from build123d import *

# Parameters (mm, degrees)
SKETCH_1_W          = 21
SKETCH_1_H          = 66
EXTRUDE_1_DEPTH     = 1.1
SKETCH_2_R          = 3
CUT_EXTRUDE_1_DEPTH = 35.647655043
SKETCH_3_W          = 21
SKETCH_3_H          = 66
SKETCH_3_W_2        = 12
SKETCH_3_H_2        = 51
EXTRUDE_2_DEPTH     = 3.9
SKETCH_4_R          = 1.9
SKETCH_4_R_2        = 1
CUT_EXTRUDE_2_DEPTH = 3
SKETCH_4_2_R        = 1
CUT_EXTRUDE_3_DEPTH = 35.989284074


with BuildPart() as part:
    # 草图1 → 凸台-拉伸1 (new body)
    with BuildSketch(Plane(origin=(0, 0, 0), x_dir=(1, 0, 0), z_dir=(0, 1, 0))):
        Rectangle(SKETCH_1_W, SKETCH_1_H)
    extrude(amount=EXTRUDE_1_DEPTH)

    # 草图2 → 切除-拉伸1 (cut, through all)
    with BuildSketch(Plane(origin=(0, 0, 0), x_dir=(-1, 0, 0), z_dir=(0, -1, 0))):
        with Locations(Location((-1.458325738, -20.003345868, 0), (0, 0, 90))):
            Circle(SKETCH_2_R)
        with Locations(Location((-1.786068296, -0.006031428, 0), (0, 0, 90))):
            Circle(SKETCH_2_R)
        with Locations(Location((-2.113810854, 19.991283012, 0), (0, 0, 90))):
            Circle(SKETCH_2_R)
    extrude(amount=-CUT_EXTRUDE_1_DEPTH, mode=Mode.SUBTRACT)

    # 草图3 → 凸台-拉伸2 (add)
    with BuildSketch(Plane(origin=(0, 1.1, 0), x_dir=(1, 0, 0), z_dir=(0, 1, 0))):
        Rectangle(SKETCH_3_W, SKETCH_3_H)
        Rectangle(SKETCH_3_W_2, SKETCH_3_H_2, mode=Mode.SUBTRACT)
    extrude(amount=EXTRUDE_2_DEPTH)

    # 草图4 → 切除-拉伸2 (cut)
    # profile 1 of 4: a face of its own
    with BuildSketch(Plane.XZ):
        with Locations(Location((0, 29.5, 0), (0, 0, 270))):
            Circle(SKETCH_4_R)
        with Locations(Location((0, 29.5, 0), (0, 0, 270))):
            Circle(SKETCH_4_R_2, mode=Mode.SUBTRACT)
    # profile 2 of 4: a face of its own
    with BuildSketch(Plane.XZ):
        with Locations(Location((-8.5, 0, 0), (0, 0, 270))):
            Circle(SKETCH_4_R)
        with Locations(Location((-8.5, 0, 0), (0, 0, 270))):
            Circle(SKETCH_4_R_2, mode=Mode.SUBTRACT)
    # profile 3 of 4: a face of its own
    with BuildSketch(Plane.XZ):
        with Locations(Location((8.5, 0, 0), (0, 0, 270))):
            Circle(SKETCH_4_R)
        with Locations(Location((8.5, 0, 0), (0, 0, 270))):
            Circle(SKETCH_4_R_2, mode=Mode.SUBTRACT)
    # profile 4 of 4: a face of its own
    with BuildSketch(Plane.XZ):
        with Locations(Location((0, -29.5, 0), (0, 0, 270))):
            Circle(SKETCH_4_R)
        with Locations(Location((0, -29.5, 0), (0, 0, 270))):
            Circle(SKETCH_4_R_2, mode=Mode.SUBTRACT)
    extrude(amount=-CUT_EXTRUDE_2_DEPTH, mode=Mode.SUBTRACT)

    # 草图4<2> → 切除-拉伸3 (cut, through all)
    with BuildSketch(Plane.XZ):
        with Locations(Location((-8.5, 0, 0), (0, 0, 270))):
            Circle(SKETCH_4_2_R)
        with Locations(Location((8.5, 0, 0), (0, 0, 270))):
            Circle(SKETCH_4_2_R)
        with Locations(Location((0, 29.5, 0), (0, 0, 270))):
            Circle(SKETCH_4_2_R)
        with Locations(Location((0, -29.5, 0), (0, 0, 270))):
            Circle(SKETCH_4_2_R)
    extrude(amount=-CUT_EXTRUDE_3_DEPTH, mode=Mode.SUBTRACT)


solid = part.part
Read the model definition and answer for the solid it produces. Units are mm, in the model's axes. A direction names the side the tool comes from. Give positions to 0.01 mm unless a question says otherwise; leave off trailing zeros. Write each loop counter-clockwise with the first axis right and the second up, starting at its lowest first coordinate (ties: lowest second). Pieces come first, ordered by that corner, then holes. Notation, with made-up numbers: (16, 70) - (20, 70) arc R23 cw to (20, 101) - close; hole circle Ø10 at (12.5, -21.75). An arc over 180 degrees is marked (long way). Use CSV: the item, a comma, the result in double quotes. Start each with the question number.
Item 1: For faces 4 (the flat face through (0, 3, -25.5)), 5 (the cylindrical face through (-0.37, 0.54, 22.38)), 6 (the flat face through (-0.82, 3, 28.68)), determine the directions among +Z, -Z, +X, -X, +Y, -Y from which every point of the face is accessible in a straight line to the end or side of a thin tool.
Item 2: The part is cut by section D-D, the plane z = 5. Give the vertices of the cut face in (x, y), and give its area (3 significant figures).
Item 3: The part is cut by section B-B, the plane y = 4.05. Give the vertices of the cut face in (x, z), and give its area (3 significant figures).
Item 4: Flat-ended cylindrical pins translate along their axes: P1, Ø6, axis at x = -1.5, z = 6.5, coming from the +Y side; P2, Ø1.9, axis at x = -8, z = -0.5, coming from the -Y side. Find the tip coordinate at first contact, or state that the pin passes through.
Item 5: The part is cut by section C-C, the plane z = 19.5. Give the vertices of the cut face in (x, y), and give its area (3 significant figures).
Item 6: Consider line 1 (X direction, y = 4.45, z = 0); line 2 (X direction, y = 4.55, z = -10); line 3 (Z direction, x = -5.5, y = 1.7). Determine where each line is inside the solid, lowest interval first.
Item 7: The mould has two halves that part along X. Classify faces 1 (the flat face through (-10.5, 2.5, 0.5)), 2 (the flat face through (0, 2, -33)), 3 (the cylindrical face through (-10.186, 1.479, -0.877)): pulls with the +X half, pulls with the -X half, needs draft (parallel to the pull), parting line crosses it, or undercut.
Item 8: The part is cut by section A-A, the plane x = 8.5. Give the vertices of the cut face in (y, z).
Taken from the geometry:
1,face 4,"+Y"
1,face 5,"+Y, -Y"
1,face 6,"-Y"
2,outline,"(-10.5, 0) - (10.5, 0) - (10.5, 5) - (6, 5) - (6, 1.1) - (-6, 1.1) - (-6, 5) - (-10.5, 5) - close"
2,area,"58.2 mm2"
3,outline,"(-10.5, -33) - (10.5, -33) - (10.5, 33) - (-10.5, 33) - close; hole circle Ø2 at (-8.5, 0); hole (-6, -25.5) - (6, -25.5) - (6, 25.5) - (-6, 25.5) - close; hole circle Ø2 at (0, -29.5); hole circle Ø2 at (0, 29.5); hole circle Ø2 at (8.5, 0)"
3,area,"761 mm2"
4,P1,"y = 1.1"
4,P2,"y = 3"
5,outline,"(-10.5, 0) - (-1.5, 0) - (-1.5, 1.1) - (-6, 1.1) - (-6, 5) - (-10.5, 5) - close; (4.42, 0) - (10.5, 0) - (10.5, 5) - (6, 5) - (6, 1.1) - (4.42, 1.1) - close"
5,area,"51.7 mm2"
6,line 1,"-10.5 to -9.5, -7.5 to -6, 6 to 7.5, 9.5 to 10.5"
6,line 2,"-10.5 to -6, 6 to 10.5"
6,line 3,"-33 to -25.5, 25.5 to 33"
7,face 1,"pulls with the -X half"
7,face 2,"needs draft"
7,face 3,"undercut"
8,outline,"(0, -33) - (5, -33) - (5, -1) - (3, -1) - (3, -1.9) - (0, -1.9) - close; (0, 1.9) - (3, 1.9) - (3, 1) - (5, 1) - (5, 33) - (0, 33) - close"
